```python
from build123d import *

# Parameters (mm, degrees)
F0_W     = 600
F0_H     = 400
F1_DEPTH = 117
F2_R     = 20
F4_DEPTH = 15
F7_DEPTH = 26
F8_W     = 570
F8_H     = 370
F9_DEPTH = 114
F9_TAPER = 3


with BuildPart() as f1:
    # F0 (on Top) → F1 (new body)
    with BuildSketch(Plane.XY):
        with Locations((8.6124254986, 0)):
            Rectangle(F0_W, F0_H)
    extrude(amount=F1_DEPTH)

    # F2
    f2_edges = [f1.edges().sort_by_distance(p)[0] for p in [
        (-291.387575, -200, 58.5),
        (308.612425, -200, 58.5),
        (308.612425, 200, 58.5),
        (-291.387575, 200, 58.5),
    ]]
    fillet(f2_edges, radius=F2_R)

    # F3 (on face) → F4 (cut)
    with BuildSketch(Plane(origin=(0, 0, 0), x_dir=(1, 0, 0), z_dir=(0, 0, -1))):
        with BuildLine():
            ThreePointArc((308.6124254986, 180), (302.7545611224, 194.1421356237), (288.6124254986, 200))
            Line((288.6124254986, 200), (-271.3875745014, 200))
            ThreePointArc((-271.3875745014, 200), (-285.5297101251, 194.1421356237), (-291.3875745014, 180))
            Line((-291.3875745014, 180), (-291.3875745014, -180))
            ThreePointArc((-291.3875745014, -180), (-285.5297101251, -194.1421356237), (-271.3875745014, -200))
            Line((-271.3875745014, -200), (288.6124254986, -200))
            ThreePointArc((288.6124254986, -200), (302.7545611224, -194.1421356237), (308.6124254986, -180))
            Line((308.6124254986, -180), (308.6124254986, 180))
        make_face()
        with BuildLine():
            ThreePointArc((-275.0983515568, 177.5), (-273.6338854627, 181.0355339059), (-270.0983515568, 182.5))
            Line((-270.0983515568, 182.5), (284.9016484432, 182.5))
            ThreePointArc((284.9016484432, 182.5), (288.4371823491, 181.0355339059), (289.9016484432, 177.5))
            Line((289.9016484432, 177.5), (289.9016484432, -177.5))
            ThreePointArc((289.9016484432, -177.5), (288.4371823491, -181.0355339059), (284.9016484432, -182.5))
            Line((284.9016484432, -182.5), (-270.0983515568, -182.5))
            ThreePointArc((-270.0983515568, -182.5), (-273.6338854627, -181.0355339059), (-275.0983515568, -177.5))
            Line((-275.0983515568, -177.5), (-275.0983515568, 177.5))
        make_face(mode=Mode.SUBTRACT)
    extrude(amount=-F4_DEPTH, mode=Mode.SUBTRACT)

    # F6 (on offset) → F7 (cut)
    with BuildSketch(Plane.XY.offset(113.5)):
        with BuildLine():
            ThreePointArc((-271.3875745014, 200), (-285.5297101251, 194.1421356237), (-291.3875745014, 180))
            Line((-291.3875745014, 180), (-291.3875745014, -180))
            ThreePointArc((-291.3875745014, -180), (-285.5297101251, -194.1421356237), (-271.3875745014, -200))
            Line((-271.3875745014, -200), (288.6124254986, -200))
            ThreePointArc((288.6124254986, -200), (302.7545611224, -194.1421356237), (308.6124254986, -180))
            Line((308.6124254986, -180), (308.6124254986, 180))
            ThreePointArc((308.6124254986, 180), (302.7545611224, 194.1421356237), (288.6124254986, 200))
            Line((288.6124254986, 200), (-271.3875745014, 200))
        make_face()
        with BuildLine():
            ThreePointArc((-278.3875745014, 180), (-276.3373219697, 184.9497474683), (-271.3875745014, 187))
            Line((-271.3875745014, 187), (288.6124254986, 187))
            ThreePointArc((288.6124254986, 187), (293.5621729669, 184.9497474683), (295.6124254986, 180))
            Line((295.6124254986, 180), (295.6124254986, -180))
            ThreePointArc((295.6124254986, -180), (293.5621729669, -184.9497474683), (288.6124254986, -187))
            Line((288.6124254986, -187), (-271.3875745014, -187))
            ThreePointArc((-271.3875745014, -187), (-276.3373219697, -184.9497474683), (-278.3875745014, -180))
            Line((-278.3875745014, -180), (-278.3875745014, 180))
        make_face(mode=Mode.SUBTRACT)
    extrude(amount=-F7_DEPTH, mode=Mode.SUBTRACT)

    # F8 (on face) → F9 (cut)
    with BuildSketch(Plane.XY.offset(117)):
        with Locations((8.6124254986, 0)):
            Rectangle(F8_W, F8_H)
    extrude(amount=-F9_DEPTH, taper=F9_TAPER, mode=Mode.SUBTRACT)


solid = f1.part
```
Check sheet for the modelled part. Datum: model origin and axes. Units: mm. A direction names the side the tool comes from. Coordinates: 2 decimals unless noted, no trailing zeros. Write item = value, one per line. Start each with the question number.
1. Thickness scan on probe 1 along X at (y, z) = (-176, 42.5); probe 2 along Z at (x, y) = (-195, -61); probe 3 along X at (y, z) = (136.5, 20.5). Record the ranges inside material, lowest first.
2. Go/stop test with flat-tipped pins: pin 1 (6 mm diameter, centred on x = 12.5, y = 158.5, fed in from +Z); pin 2 (8 mm diameter, centred on y = -73.5, z = 95.5, fed in from -X); pin 3 (21 mm diameter, centred on y = 57, z = 98.5, fed in from +X). Record where each tip stops, or that it passes through.
3. Tool access check on faces 5 (the flat face through (3, 3, 0)), 6 (the flat face through (5, 187, 101)), 7 (the flat face through (4, -182.5, 7)), 8 (the flat face through (11, 182.5, 7)), 9 (the flat face through (-275.098, 2, 7)). Record the directions out of +Z, -Z, +X, -X, +Y, -Y that give a thin tool (end or side, any length) a straight path to the whole face; none if there is none.
4. Mould release check, pull along Z, two halves, no side actions. Record for faces 1 (the flat face through (289.902, -2, 7)), 2 (the flat face through (-15, 192, 15)), 3 (the flat face through (13, -187, 101)), 4 (the flat face through (-15, -192, 113.5)): pulls with the +Z half, pulls with the -Z half, needs draft (parallel to the pull), parting line crosses it, or undercut.
The answers:
q1.probe_1 = -291.39 to -272.48, 289.71 to 308.61
q1.probe_2 = 0 to 3
q1.probe_3 = -291.39 to -271.33, 288.56 to 308.61
q2.pin_1 = 3
q2.pin_2 = -278.39
q2.pin_3 = 295.61
q3.face_5 = -Z, +X, -X, +Y, -Y
q3.face_6 = +X, -X, +Y
q3.face_7 = -Z, +X, -X, -Y
q3.face_8 = -Z, +X, -X, +Y
q3.face_9 = -Z, -X, +Y, -Y
q4.face_1 = needs draft
q4.face_2 = pulls with the -Z half
q4.face_3 = undercut
q4.face_4 = undercut
